Check sheet for the modelled part. Datum: model origin and axes. Units: mm. Face numbers are marked on the shaded views. Round coordinates to 2 decimals unless told otherwise and drop trailing zeros. Write each loop counter-clockwise with the first axis right and the second up, starting at its lowest first coordinate (ties: lowest second). Pieces come first, ordered by that corner, then holes.
Item 1: Section check B-B, the plane x = -3.5. Record the cut outline in (y, z), plus the area to 3 significant figures.
Item 2: Release check for a two-part mould opening along X. For the marked faces 1 and 2 record: pulls with the +X half, pulls with the -X half, needs draft (parallel to the pull), parting line crosses it, or undercut.
Item 3: Material ranges on line 1 along Y through (x, z) = (-33.02, 3.4); line 2 along X through (y, z) = (0, 2.5); line 3 along X through (y, z) = (-2.5, 3), recorded low to high.
Item 4: Section check C-C, the plane x = 33.02. Record the cut outline in (y, z).
Item 5: Section check D-D, the plane y = 0. State how many separate pieces and enclosed holes the cut face has, plus the area to 3 significant figures.
Item 6: Depth check by flat-ended pin: pin 1 (3 mm diameter, centred on x = 1.5, y = -7, fed in from +Z); pin 2 (4 mm diameter, centred on x = -19.5, y = -4, fed in from +Z); pin 3 (2 mm diameter, centred on y = 5.5, z = 6, fed in from +X). Enter the tip coordinate at first touch or a pass-through.
Item 7: Section check A-A, the plane x = -33.02. Record the cut outline in (y, z).
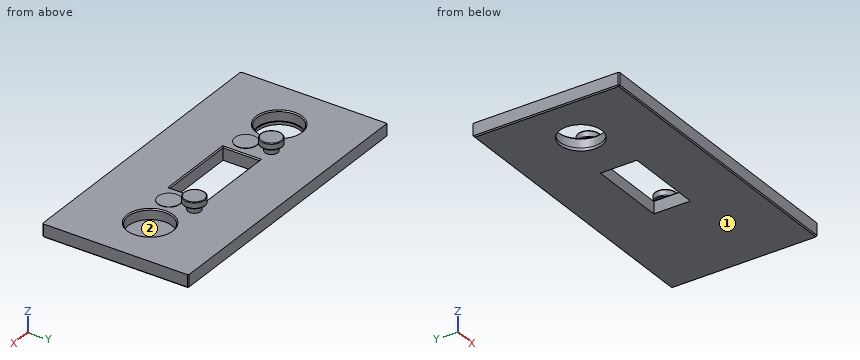
from build123d import *

# Parameters (mm, degrees)
F0_W     = 101.6
F0_H     = 50.8
F0_R     = 7.62
F0_R_2   = 3.81
F0_W_2   = 27.305
F0_H_2   = 12.7
F0_R_3   = 2.2225
F1_DEPTH = 4.572
F0_R_4   = 7.3025
F2_DEPTH = 1.016
F0_R_5   = 2.2174229623
F3_DEPTH = 6.858
F4_DEPTH = 4.6736
F5_R     = 3.683
F5_R_2   = 2.2225
F6_DEPTH = 2.286
F7_R     = 0.254
F8_SIZE  = 0.381


with BuildPart() as f1:
    # F0 (on Top) → F1 (new body)
    with BuildSketch(Plane.XY):
        Rectangle(F0_W, F0_H)
        with Locations((-33.02, 0)):
            Circle(F0_R, mode=Mode.SUBTRACT)
        with Locations((-19.685, -2.54)):
            Circle(F0_R_2, mode=Mode.SUBTRACT)
        Rectangle(F0_W_2, F0_H_2, mode=Mode.SUBTRACT)
        with Locations((19.685, -2.54)):
            Circle(F0_R_2, mode=Mode.SUBTRACT)
        with Locations((33.02, 0)):
            Circle(F0_R, mode=Mode.SUBTRACT)
        with Locations((-19.685, 6.35)):
            Circle(F0_R_3, mode=Mode.SUBTRACT)
        with Locations((19.685, 6.35)):
            Circle(F0_R_3, mode=Mode.SUBTRACT)
    extrude(amount=F1_DEPTH)

    # F0 (on Top) → F2 (join)
    with BuildSketch(Plane.XY):
        Rectangle(F0_W, F0_H)
        with Locations((-33.02, 0)):
            Circle(F0_R, mode=Mode.SUBTRACT)
        with Locations((-19.685, -2.54)):
            Circle(F0_R_2, mode=Mode.SUBTRACT)
        Rectangle(F0_W_2, F0_H_2, mode=Mode.SUBTRACT)
        with Locations((19.685, -2.54)):
            Circle(F0_R_2, mode=Mode.SUBTRACT)
        with Locations((33.02, 0)):
            Circle(F0_R, mode=Mode.SUBTRACT)
        with Locations((-19.685, 6.35)):
            Circle(F0_R_3, mode=Mode.SUBTRACT)
        with Locations((19.685, 6.35)):
            Circle(F0_R_3, mode=Mode.SUBTRACT)
        with Locations((33.02, 0)):
            Circle(F0_R)
        with Locations((-33.02, 0)):
            Circle(F0_R)
        with Locations((-33.02, 0)):
            Circle(F0_R_4, mode=Mode.SUBTRACT)
    extrude(amount=F2_DEPTH)

    # F0 (on Top) → F3 (join)
    with BuildSketch(Plane.XY):
        with Locations((19.685, 6.35)):
            Circle(F0_R_3)
        with Locations((19.685, 6.35)):
            Circle(F0_R_5, mode=Mode.SUBTRACT)
        with Locations((19.685, 6.35)):
            Circle(F0_R_5)
        with Locations((-19.685, 6.35)):
            Circle(F0_R_3)
    extrude(amount=F3_DEPTH)

    # F0 (on Top) → F4 (join)
    with BuildSketch(Plane.XY):
        with Locations((-19.685, -2.54)):
            Circle(F0_R_2)
        with Locations((19.685, -2.54)):
            Circle(F0_R_2)
    extrude(amount=F4_DEPTH)

    # F5 (on face) → F6 (join)
    with BuildSketch(Plane.XY.offset(6.858)):
        with Locations((19.685, 6.35)):
            Circle(F5_R)
        with Locations((19.685, 6.35)):
            Circle(F5_R_2, mode=Mode.SUBTRACT)
        with Locations((-19.685, 6.35)):
            Circle(F5_R)
        with Locations((19.685, 6.35)):
            Circle(F5_R_2)
    extrude(amount=F6_DEPTH)

    # F7
    f7_edges = [f1.edges().sort_by_distance(p)[0] for p in [
        (-23.368, 6.35, 9.144),
        (-16.002, 6.35, 8.001),
        (-23.368, 6.35, 6.858),
        (16.002, 6.35, 9.144),
        (16.002, 6.35, 6.858),
    ]]
    fillet(f7_edges, radius=F7_R)

    # F8
    f8_edges = [f1.edges().sort_by_distance(p)[0] for p in [
        (25.4, 0, 4.572),
        (-40.64, 0, 4.572),
        (50.8, 25.4, 2.286),
        (0, 25.4, 0),
        (50.8, 0, 0),
        (50.8, -25.4, 2.286),
        (0, -25.4, 0),
        (-50.8, -25.4, 2.286),
        (-50.8, 0, 0),
        (0, 6.35, 4.572),
        (-13.6525, 0, 4.572),
        (0, -6.35, 4.572),
        (13.6525, 0, 4.572),
    ]]
    chamfer(f8_edges, length=F8_SIZE)


solid = f1.part
Values found:
1. outline: (-25.4, 0.38) - (-25.02, 0) - (-6.35, 0) - (-6.35, 4.19) - (-6.73, 4.57) - (-25.4, 4.57) - close; (6.35, 0) - (25.02, 0) - (25.4, 0.38) - (25.4, 4.57) - (6.73, 4.57) - (6.35, 4.19) - close
1. area: 174 mm2
2. face 1: needs draft
2. face 2: undercut
3. line 1: y = -25.4 to -7.62, 7.62 to 25.4
3. line 2: x = -50.8 to -40.64, -25.4 to -13.65, 13.65 to 25.4, 40.64 to 50.8
3. line 3: x = -50.8 to -40.22, -25.82 to -13.65, 13.65 to 25.82, 40.22 to 50.8
4. outline: (-25.4, 0.38) - (-25.02, 0) - (25.02, 0) - (25.4, 0.38) - (25.4, 4.57) - (8, 4.57) - (7.62, 4.19) - (7.62, 1.02) - (-7.62, 1.02) - (-7.62, 4.19) - (-8, 4.57) - (-25.4, 4.57) - close
5. separate pieces: 3
5. enclosed holes: 0
5. area: 217 mm2
6. pin 1: stops at z = 4.57
6. pin 2: stops at z = 4.67
6. pin 3: stops at x = 23.27
7. outline: (-25.4, 0.38) - (-25.02, 0) - (-7.3, 0) - (-7.3, 1.02) - (-7.62, 1.02) - (-7.62, 4.19) - (-8, 4.57) - (-25.4, 4.57) - close; (7.3, 0) - (25.02, 0) - (25.4, 0.38) - (25.4, 4.57) - (8, 4.57) - (7.62, 4.19) - (7.62, 1.02) - (7.3, 1.02) - close
